Here's how the part is built. I have some questions about the finished solid (model axes, mm). Face numbers are marked on the shaded views. Give positions to 0.01 mm unless a question says otherwise; leave off trailing zeros. Loops run counter-clockwise (first coordinate to the right, second up) from the corner with the lowest first, then second, coordinate; pieces in that order, holes last.
Q1. Thinking about a two-plate mould opening in Z: for the marked faces 1 and 2, which applies, pulls with the +Z half, pulls with the -Z half, needs draft (parallel to the pull), parting line crosses it, or undercut?
Q2. Suppose I cut it at B-B (y = 6.5). List the corners of the cut face in (x, z) for me.
Q3. I need wall thicknesses on probe 1 along Y at (x, z) = (-1.3, 0); probe 2 along Z at (x, y) = (-0.1, -78.5); probe 3 along Z at (x, y) = (-1.75, 90). Which ranges of each line are inside material? Lowest first, please.
Q4. Suppose I cut it at C-C (z = -5.5). List the corners of the cut face in (x, y) for me, and give its area (3 significant figures).
Q5. Suppose I cut it at A-A (x = -0.1). List the corners of the cut face in (y, z) for me, and give its area (3 significant figures).
Q6. I'm going to push a flat-ended pin straight in: P1, Ø3, axis at y = 67, z = 4, coming from the +X side. Where does the tip first touch, or does it pass through?
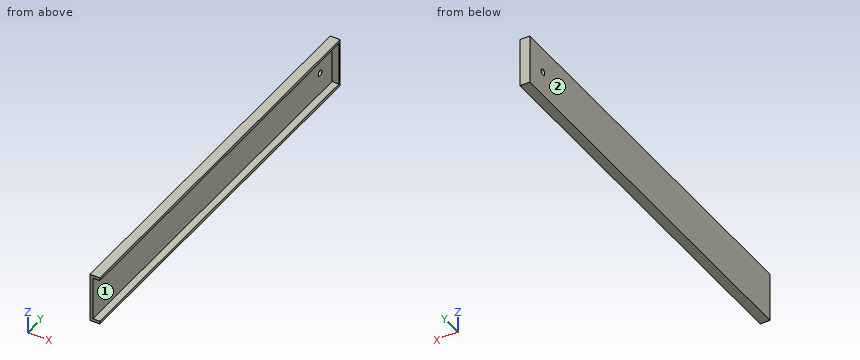
```python
from build123d import *

# Parameters (mm, degrees)
BOSS_EXTRUDE1_DEPTH = 100
BOSS_EXTRUDE2_START = 100
SKETCH1_3_W         = 3.5
SKETCH1_3_H         = 22
BOSS_EXTRUDE2_DEPTH = 1
SKETCH2_R           = 1.5
CUT_EXTRUDE1_DEPTH  = 25


with BuildPart() as part:
    # Sketch1 → Boss-Extrude1 (new, symmetric)
    with BuildSketch(Plane(origin=(0, 0, 0), x_dir=(1, 0, 0), z_dir=(0, 1, 0))):
        Polygon((-2.5, -12.5), (-2.5, 12.5), (2.5, 12.5), (2.5, 11), (-1, 11), (-1, -11), (2.5, -11), (2.5, -12.5), align=None)
    extrude(amount=BOSS_EXTRUDE1_DEPTH, both=True)

    # Sketch1<3> → Boss-Extrude2 (add)
    with BuildSketch(Plane(origin=(0, 0, 0), x_dir=(1, 0, 0), z_dir=(0, 1, 0)).offset(BOSS_EXTRUDE2_START)):
        with Locations((0.75, 0)):
            Rectangle(SKETCH1_3_W, SKETCH1_3_H)
        Polygon((2.5, 11), (-1, 11), (-1, -11), (2.5, -11), (2.5, -12.5), (-2.5, -12.5), (-2.5, 12.5), (2.5, 12.5), align=None)
    extrude(amount=BOSS_EXTRUDE2_DEPTH)

    # Sketch2 → Cut-Extrude1 (cut)
    with BuildSketch(Plane(origin=(-1, 0, 0), x_dir=(0, 0, -1), z_dir=(1, 0, 0))):
        with Locations((0, 90)):
            Circle(SKETCH2_R)
    extrude(amount=-CUT_EXTRUDE1_DEPTH, mode=Mode.SUBTRACT)


solid = part.part
```
Solutions:
1. face 1: undercut
1. face 2: needs draft
2. outline: (-2.5, -12.5) - (2.5, -12.5) - (2.5, -11) - (-1, -11) - (-1, 11) - (2.5, 11) - (2.5, 12.5) - (-2.5, 12.5) - close
3. probe 1: y = -100 to 88.5, 91.5 to 101
3. probe 2: z = -12.5 to -11, 11 to 12.5
3. probe 3: z = -12.5 to -1.5, 1.5 to 12.5
4. outline: (-2.5, -100) - (-1, -100) - (-1, 100) - (2.5, 100) - (2.5, 101) - (-2.5, 101) - close
4. area: 305 mm2
5. outline: (-100, -12.5) - (101, -12.5) - (101, 12.5) - (-100, 12.5) - (-100, 11) - (100, 11) - (100, -11) - (-100, -11) - close
5. area: 625 mm2
6. P1: stops at x = -1
